Verification items for the finished model (mm, model axes). A direction names the side the tool comes from. Give positions to 0.01 mm unless a question says otherwise; leave off trailing zeros. Loops run counter-clockwise (first coordinate to the right, second up) from the corner with the lowest first, then second, coordinate; pieces in that order, holes last. Notation, with made-up numbers: M 73,0 L 99,0 A25 ccw 99,32 Z; hole C 78.25,33 d5. An arc over 180 degrees is marked long. Answer in a Markdown table with one row per item.
```python
from build123d import *

# Parameters (mm, degrees)
ESBO_O4_W                        = 2.25
ESBO_O4_H                        = 16
F_4_5_4_5_DIAMETER_HOLE2_D       = 4.5
F_4_5_4_5_DIAMETER_HOLE2_DEPTH   = 18
F_4_5_4_5_DIAMETER_HOLE2_TIP     = 1.351936393
ESBO_O12_R                       = 16
ESBO_O12_R_2                     = 9
RESSALTO_EXTRUS_O1_DEPTH         = 1
CHANFRO1_SIZE                    = 0.5
CHANFRO2_SIZE                    = 0.25
FURO_DE_DI_METRO_4_5_4_5_2_D     = 4.5
FURO_DE_DI_METRO_4_5_4_5_2_DEPTH = 8
FURO_DE_DI_METRO_4_5_4_5_2_TIP   = 1.351936393
CORTE_EXTRUS_O4_START            = -0.5
ESBO_O18_R                       = 4
ESBO_O18_R_2                     = 2.25
CORTE_EXTRUS_O4_DEPTH            = 0.5
PADR_OCIRCULAR6_COUNT            = 2
PADR_OCIRCULAR6_ANGLE            = 30
PADR_OCIRCULAR7_COUNT            = 2
PADR_OCIRCULAR7_ANGLE            = 210


# Read off the part's stored shape, not the designer's step: PadrãoCircular5
with BuildPart() as part:
    # Esboço1 → Revolução1 (revolve)
    with BuildSketch(Plane.XY, mode=Mode.PRIVATE) as revolu_o1_sk:
        Polygon((3, -9), (16, -9), (16, 5), (9, 5), (9, -5), (3, -5), align=None)
    revolve(revolu_o1_sk.sketch.rotate(Axis((0, -9, 0), (0, 1, 0)), 90), axis=Axis((0, -9, 0), (0, 1, 0)))

    # Esboço4 → Furo de diâmetro Ø4.5 (4.5)1 (revolve, cut)
    with BuildSketch(Plane(origin=(16, 0, 0), x_dir=(0, 0, -1), z_dir=(0, 1, 0))):
        with Locations((1.125, 8)):
            Rectangle(ESBO_O4_W, ESBO_O4_H)
    revolve(axis=Axis((22.35, 0, 0), (-1, 0, 0)), mode=Mode.SUBTRACT)

    # Ø4.5 (4.5) Diameter Hole2
    with Locations(Plane(origin=(-13.856406461, 0, -8), x_dir=(0, -1, 0), z_dir=(-0.8660254037844364, 0, -0.5000000000000041))):
        with Locations((0, 0)):
            Hole(F_4_5_4_5_DIAMETER_HOLE2_D / 2, depth=F_4_5_4_5_DIAMETER_HOLE2_DEPTH)
            with Locations((0, 0, -(F_4_5_4_5_DIAMETER_HOLE2_DEPTH + F_4_5_4_5_DIAMETER_HOLE2_TIP / 2))):  # 118° drill point
                Cone(0, F_4_5_4_5_DIAMETER_HOLE2_D / 2, F_4_5_4_5_DIAMETER_HOLE2_TIP, mode=Mode.SUBTRACT)

    # Esboço12 → Ressalto-extrusão1 (add)
    with BuildSketch(Plane(origin=(0, 5, 0), x_dir=(1, 0, 0), z_dir=(0, 1, 0))):
        with Locations(Location((0, 0, 0), (0, 0, 90))):
            Circle(ESBO_O12_R)
        with Locations(Location((0, 0, 0), (0, 0, 90))):
            Circle(ESBO_O12_R_2, mode=Mode.SUBTRACT)
    extrude(amount=RESSALTO_EXTRUS_O1_DEPTH)

    # Esboço13 → Furo roscado de M3x0.51 (revolve, cut)
    with BuildSketch(Plane(origin=(11.328847338, 6, -5.282728272), x_dir=(0, 0, 1), z_dir=(1, 0, 0))):
        Polygon((0, 0), (0, 10.751075774), (1.25, 10), (1.25, 0), align=None)
    revolve(axis=Axis((11.328847338, 12.35, -5.282728272), (0, -1, 0)), mode=Mode.SUBTRACT)

    # PadrãoCircular5 outline → PadrãoCircular5 (revolve, cut)
    with BuildSketch(Plane(origin=(5.282728272, 0, 11.328847338), x_dir=(1, 0, 0), z_dir=(0, 0, 1))):
        Polygon((0, 6), (0, -4.751075774), (1.25, -4), (1.25, 6), align=None)
    revolve(axis=Axis((5.282728272, 0, 11.328847338), (0, 1, 0)), mode=Mode.SUBTRACT)

    # Padr_oCircular5 2 outline → Padr_oCircular5 2 (revolve, cut)
    with BuildSketch(Plane(origin=(-11.328847338, 0, 5.282728272), x_dir=(1, 0, 0), z_dir=(0, 0, 1))):
        Polygon((0, 6), (0, -4.751075774), (1.25, -4), (1.25, 6), align=None)
    revolve(axis=Axis((-11.328847338, 0, 5.282728272), (0, 1, 0)), mode=Mode.SUBTRACT)

    # Padr_oCircular5 3 outline → Padr_oCircular5 3 (revolve, cut)
    with BuildSketch(Plane(origin=(-5.282728272, 0, -11.328847338), x_dir=(1, 0, 0), z_dir=(0, 0, 1))):
        Polygon((0, 6), (0, -4.751075774), (1.25, -4), (1.25, 6), align=None)
    revolve(axis=Axis((-5.282728272, 0, -11.328847338), (0, 1, 0)), mode=Mode.SUBTRACT)

    # Chanfro1
    chanfro1_edges = [part.edges().sort_by_distance(p)[0] for p in [
        (0, -5, 3),
    ]]
    chamfer(chanfro1_edges, length=CHANFRO1_SIZE)

    # Chanfro2
    chanfro2_edges = [part.edges().sort_by_distance(p)[0] for p in [
        (0, 6, 9),
    ]]
    chamfer(chanfro2_edges, length=CHANFRO2_SIZE)

    # Furo de diâmetro Ø4.5 (4.5)2
    with Locations(Plane(origin=(-16, 0, 0), x_dir=(0, 0, -1), z_dir=(-1, 0, 0))):
        with Locations((0, 0)):
            Hole(FURO_DE_DI_METRO_4_5_4_5_2_D / 2, depth=FURO_DE_DI_METRO_4_5_4_5_2_DEPTH)
            with Locations((0, 0, -(FURO_DE_DI_METRO_4_5_4_5_2_DEPTH + FURO_DE_DI_METRO_4_5_4_5_2_TIP / 2))):  # 118° drill point
                Cone(0, FURO_DE_DI_METRO_4_5_4_5_2_D / 2, FURO_DE_DI_METRO_4_5_4_5_2_TIP, mode=Mode.SUBTRACT)

    # Esboço18 → Corte-extrusão4 (cut)
    with BuildSketch(Plane(origin=(-13.856406461, 0, -8), x_dir=(0, -1, 0), z_dir=(-0.8660254037844364, 0, -0.5000000000000041)).offset(CORTE_EXTRUS_O4_START)):
        Circle(ESBO_O18_R)
        with Locations(Location((0, 0, 0), (0, 0, 90))):
            Circle(ESBO_O18_R_2, mode=Mode.SUBTRACT)
    corte_extrus_o4 = extrude(amount=CORTE_EXTRUS_O4_DEPTH, mode=Mode.SUBTRACT)

    # PadrãoCircular6: Corte-extrusão4 ×2 about axis
    padr_ocircular6_axis = Axis((0, -9.75, 0), (0, 1, 0))
    for i in range(1, PADR_OCIRCULAR6_COUNT):
        add(corte_extrus_o4.rotate(padr_ocircular6_axis, i * PADR_OCIRCULAR6_ANGLE / (PADR_OCIRCULAR6_COUNT - 1)), mode=Mode.SUBTRACT)

    # PadrãoCircular7: Corte-extrusão4 ×2 about axis
    padr_ocircular7_axis = Axis((0, -9.75, 0), (0, 1, 0))
    for i in range(1, PADR_OCIRCULAR7_COUNT):
        add(corte_extrus_o4.rotate(padr_ocircular7_axis, i * PADR_OCIRCULAR7_ANGLE / (PADR_OCIRCULAR7_COUNT - 1)), mode=Mode.SUBTRACT)


solid = part.part
```
Item 1: Sectioned sample at D-D (y = -8). Record the cut outline in (x, z).
Reported:
| item | result |
|---|---|
| outline | C 0,0 d32; hole C 0,0 d6 |
Item 2: Go/stop test with flat-tipped pins: pin 1 (4 mm diameter, centred on y = 0, z = 0, fed in from +X); pin 2 (5.5 mm diameter, centred on x = 3.5, z = 0, fed in from +Y); pin 3 (5 mm diameter, centred on x = 11.5, y = -2.5, fed in from +Z); pin 4 (6 mm diameter, centred on y = 0.5, z = 5.5, fed in from -X). Record where each tip stops, or that it passes through.
Reported:
| item | result |
|---|---|
| pin 1 | passes through |
| pin 2 | stops at y = -5 |
| pin 3 | stops at z = 13.23 |
| pin 4 | stops at x = -15.68 |
Item 3: Sectioned sample at B-B (x = 0). Record the cut outline in (y, z), and give its area (3 significant figures).
Reported:
| item | result |
|---|---|
| outline | M -9,-16 L 6,-16 L 6,-9.25 L 5.75,-9 L -5,-9 L -5,-3.5 L -5.5,-3 L -9,-3 Z; M -9,3 L -5.5,3 L -5,3.5 L -5,9 L 5.75,9 L 6,9.25 L 6,16 L -9,16 Z |
| area | 258 mm^2 |
Item 4: Scan lines: L1, parallel to X at y = 2.5, z = -4.5; L2, parallel to X at y = -2.5, z = -5.5; L3, parallel to Z at x = -5, y = -3. Record each from-to range of solid material in increasing order. Write a range as [from, to].
Reported:
| item | result |
|---|---|
| L1 | x = [-15.35, -7.79], [7.79, 10.35], [12.3, 15.35] |
| L2 | x = [-14.72, -7.12], [7.12, 10.1], [12.56, 15.02] |
| L3 | z = [-15.2, -12.55], [-10.11, -7.48], [7.48, 15.2] |
Item 5: Release check for a two-part mould opening along Z. For faces 1 (the flat face through (-0.2, -9, 3.3)), 2 (the cylindrical face through (5.12, 1.07, 10.09)) record: released by +Z, released by -Z, zero draft, split by the parting line, or undercut.
Reported:
| item | result |
|---|---|
| face 1 | zero draft |
| face 2 | undercut |
Item 6: Tool access check on faces 3 (the cylindrical face through (-5.554, 1.07, -10.109)), 4 (the cylindrical face through (-13.6, 4, -7.8)), 5 (the cylindrical face through (-15.7, -4, -0.1)). Record the directions out of +Z, -Z, +X, -X, +Y, -Y that give a thin tool (end or side, any length) a straight path to the whole face; none if there is none.
Reported:
| item | result |
|---|---|
| face 3 | +Y |
| face 4 | none |
| face 5 | -X |
Item 7: Sectioned sample at C-C (y = 0). Record the cut outline in (x, z).
Reported:
| item | result |
|---|---|
| outline | M -15.5,-3.97 A16 ccw -15.41,-4.31 L -14.55,-5.8 L -8.67,-2.41 A9 cw -8.71,-2.25 L -15.5,-2.25 Z; M -15.5,2.25 L -8.71,2.25 A9 cw 8.71,2.25 L 15.5,2.25 L 15.5,3.97 A16 ccw -15.5,3.97 Z; M -12.3,-9.7 L -11.44,-11.19 A16 ccw 15.5,-3.97 L 15.5,-2.25 L 8.71,-2.25 A9 cw -6.42,-6.31 Z; hole C -11.33,5.28 d2.5; hole C -5.28,-11.33 d2.5; hole C 5.28,11.33 d2.5; hole C 11.33,-5.28 d2.5 |
Item 8: Sectioned sample at A-A (z = 0). State how many separate pieces and enclosed holes the cut face has, and give its area (3 significant figures).
Reported:
| item | result |
|---|---|
| separate pieces | 4 |
| enclosed holes | 0 |
| area | 191 mm^2 |
